Geometry: final body of the model. Coordinates: model frame, mm. A direction names the side the tool comes from. Give positions to 0.01 mm unless a question says otherwise; leave off trailing zeros. Loops run counter-clockwise (first coordinate to the right, second up) from the corner with the lowest first, then second, coordinate; pieces in that order, holes last.
1. Material intervals for line 1 along Y through (x, z) = (23.75, -26.9); line 2 along X through (y, z) = (-2.95, 23.75); line 3 along X through (y, z) = (63, -28), sorted ascending.
2. Draft query along Z for faces 1 (the face through (-30, 18, -28)), 2 (the face through (25.52, -2.46, 24.88)), 3 (the face through (25.52, -2.46, -22.62)), 4 (the face through (0, 37, -25)). Return one class per face: +Z half, -Z half, draft (parallel to the pull), parting line (faces both ways), or undercut.
3. Section C-C, the plane x = 23.75. Output: boundary loops of the cut face in (y, z).
4. Access query for faces 5 (the face through (22, 26.25, -28)), 6 (the face through (-16.25, -2, 28)), 7 (the face through (-22, 53.75, -28)), 8 (the face through (15, -2, -19.5)), 9 (the face through (-30, -2, 0)). Directions: +Z, -Z, +X, -X, +Y, -Y. A direction counts if a zero-diameter tool reaches every point of the face in a straight line with its end or side. Return the directions, or none.
5. Section B-B, the plane z = 23.75. Output: boundary loops of the cut face in (x, y).
6. Section D-D, the plane x = -20. Output: boundary loops of the cut face in (y, z).
7. First-contact query: P1, Ø2, axis at x = 16, y = 34.5, coming from the -Z side; P2, Ø4, axis at x = -4.5, y = -3.5, coming from the +Z side; P3, Ø5.5, axis at y = 36, z = -28.5, coming from the +X side; P4, Ø0.8, axis at x = -15.5, y = -2.5, coming from the -Z side. Flat tips, straight axial feed; report the tip coordinate or a pass-through.
8. Section A-A, the plane y = 50. Output: boundary loops of the cut face in (x, z).
from build123d import *

# Parameters (mm, degrees)
SKETCH_1_R                        = 2.1
SM_BASE_FLANGE_1_DEPTH            = 5
SM_EDGE_FLANGE_1_STRIP_W          = 26
SM_EDGE_FLANGE_1_STRIP_H          = 5
SM_EDGE_FLANGE_1_STRIP_CUT_DEPTH  = 27.5
SM_EDGE_FLANGE_1_RELIEF_W         = 28.5
SM_EDGE_FLANGE_1_RELIEF_H         = 2.5
SM_EDGE_FLANGE_1_RELIEF_CUT_DEPTH = 5
SM_EDGE_FLANGE_1_DEPTH            = 27.5
EXTRUDE_START                     = -30
SKETCH_9_W                        = 16.25
SKETCH_9_H                        = 16.25
EXTRUDE_1_DEPTH                   = 5
CUT_EXTRUDE_START                 = -30
SKETCH_10_R                       = 2.5
CUT_EXTRUDE_1_DEPTH               = 5
SKETCH_11_R                       = 2.1
CUT_EXTRUDE_2_DEPTH               = 5


# Sheet-metal steps are written as plain solids
with BuildPart() as part:
    # Sketch 1 → 基体-法兰1 (new body)
    with BuildSketch(Plane(origin=(0, 0, 0), x_dir=(1, 0, 0), z_dir=(0, 1, 0))):
        Polygon((-16.25, 25), (-16.25, 30), (-30, 30), (-30, -30), (-16.25, -30), (-16.25, -25), (16.25, -25), (16.25, -30), (30, -30), (30, 30), (16.25, 30), (16.25, 25), align=None)
        with Locations(Location((-23.75, 23.75, 0), (0, 0, 270))):
            Circle(SKETCH_1_R, mode=Mode.SUBTRACT)
        with Locations(Location((23.75, 23.75, 0), (0, 0, 270))):
            Circle(SKETCH_1_R, mode=Mode.SUBTRACT)
        with Locations(Location((-23.75, -23.75, 0), (0, 0, 270))):
            Circle(SKETCH_1_R, mode=Mode.SUBTRACT)
        with Locations(Location((23.75, -23.75, 0), (0, 0, 270))):
            Circle(SKETCH_1_R, mode=Mode.SUBTRACT)
    extrude(amount=-SM_BASE_FLANGE_1_DEPTH)

    # 边线-法兰1 strip (across the edge) → 边线-法兰1 strip cut (cut)
    with BuildSketch(Plane(origin=(13.75, 0, -25), x_dir=(0, 0, 1), z_dir=(-1, 0, 0))):
        with Locations((-10, -2.5)):
            Rectangle(SM_EDGE_FLANGE_1_STRIP_W, SM_EDGE_FLANGE_1_STRIP_H)
    extrude(amount=SM_EDGE_FLANGE_1_STRIP_CUT_DEPTH, mode=Mode.SUBTRACT)

    # 边线-法兰1 relief (on the sheet) → 边线-法兰1 relief cut (cut)
    with BuildSketch(Plane(origin=(13.75, 0, -22), x_dir=(0, 0, 1), z_dir=(0, 1, 0))):
        with Locations((-11.75, 1.25)):
            Rectangle(SM_EDGE_FLANGE_1_RELIEF_W, SM_EDGE_FLANGE_1_RELIEF_H)
        with Locations((-11.75, -28.75)):
            Rectangle(SM_EDGE_FLANGE_1_RELIEF_W, SM_EDGE_FLANGE_1_RELIEF_H)
    extrude(amount=-SM_EDGE_FLANGE_1_RELIEF_CUT_DEPTH, mode=Mode.SUBTRACT)

    # 边线-法兰1 section (across the edge) → 边线-法兰1 (add)
    with BuildSketch(Plane(origin=(13.75, 0, -25), x_dir=(0, 0, 1), z_dir=(-1, 0, 0))):
        with BuildLine():
            Line((-5, 3), (-5, 70))
            Line((-5, 70), (0, 70))
            Line((0, 70), (0, 3))
            ThreePointArc((0, 3), (0.878679656, 0.878679656), (3, 0))
            Line((3, 0), (3, -5))
            ThreePointArc((3, -5), (-2.656854249, -2.656854249), (-5, 3))
        make_face()
    extrude(amount=SM_EDGE_FLANGE_1_DEPTH)

    # 草图9 → 凸台-拉伸1 (add)
    with BuildSketch(Plane.XY.offset(EXTRUDE_START)):
        with Locations((-21.875, 61.875)):
            Rectangle(SKETCH_9_W, SKETCH_9_H)
        with Locations((21.875, 61.875)):
            Rectangle(SKETCH_9_W, SKETCH_9_H)
        with Locations((-21.875, 18.125)):
            Rectangle(SKETCH_9_W, SKETCH_9_H)
        with Locations((21.875, 18.125)):
            Rectangle(SKETCH_9_W, SKETCH_9_H)
    extrude(amount=EXTRUDE_1_DEPTH)

    # 草图10 → 切除-拉伸1 (cut)
    with BuildSketch(Plane.XY.offset(CUT_EXTRUDE_START)):
        with Locations(Location((0, 50, 0), (0, 0, 90))):
            Circle(SKETCH_10_R)
        with Locations(Location((0, 30, 0), (0, 0, 90))):
            Circle(SKETCH_10_R)
    extrude(amount=CUT_EXTRUDE_1_DEPTH, mode=Mode.SUBTRACT)

    # 草图11 → 切除-拉伸2 (cut)
    with BuildSketch(Plane.XY.offset(CUT_EXTRUDE_START)):
        with Locations((-23.75, 16.25)):
            Circle(SKETCH_11_R)
        with Locations((-23.75, 63.75)):
            Circle(SKETCH_11_R)
        with Locations((23.75, 63.75)):
            Circle(SKETCH_11_R)
        with Locations((23.75, 16.25)):
            Circle(SKETCH_11_R)
    extrude(amount=CUT_EXTRUDE_2_DEPTH, mode=Mode.SUBTRACT)


solid = part.part
Answers below:
1. line 1: y = -5 to 0, 10 to 14.15, 18.35 to 26.25, 53.75 to 61.65, 65.85 to 70
1. line 2: x = -30 to -25.85, -21.65 to 21.65, 25.85 to 30
1. line 3: x = -30 to -25.71, -21.79 to 21.79, 25.71 to 30
2. face 1: draft
2. face 2: undercut
2. face 3: undercut
2. face 4: +Z half
3. outline: (-5, -30) - (0, -30) - (0, -25.85) - (-5, -25.85) - close; (-5, -21.65) - (0, -21.65) - (0, 21.65) - (-5, 21.65) - close; (-5, 25.85) - (0, 25.85) - (0, 30) - (-5, 30) - close; (10, -30) - (14.15, -30) - (14.15, -25) - (10, -25) - close; (18.35, -30) - (26.25, -30) - (26.25, -25) - (18.35, -25) - close; (53.75, -30) - (61.65, -30) - (61.65, -25) - (53.75, -25) - close; (65.85, -30) - (70, -30) - (70, -25) - (65.85, -25) - close
4. face 5: +Z, -Z, +X
4. face 6: +Z, +Y, -Y
4. face 7: +Z, -Z, -X
4. face 8: -Z, +Y, -Y
4. face 9: +Z, -Z, -X, +Y, -Y
5. outline: (-30, -5) - (-25.85, -5) - (-25.85, 0) - (-30, 0) - close; (-21.65, -5) - (21.65, -5) - (21.65, 0) - (-21.65, 0) - close; (25.85, -5) - (30, -5) - (30, 0) - (25.85, 0) - close
6. outline: (-5, -30) - (0, -30) - (0, 30) - (-5, 30) - close; (10, -30) - (26.25, -30) - (26.25, -25) - (10, -25) - close; (53.75, -30) - (70, -30) - (70, -25) - (53.75, -25) - close
7. P1: passes through
7. P2: stops at z = 25
7. P3: stops at x = 13.75
7. P4: stops at z = -19.5
8. outline: (-13.75, -30) - (-2.5, -30) - (-2.5, -25) - (-13.75, -25) - close; (2.5, -30) - (13.75, -30) - (13.75, -25) - (2.5, -25) - close
